from build123d import *

# Parameters (mm, degrees)
SKETCH_R        = 2.25
SKETCH_R_2      = 11.25
SKETCH_R_3      = 1.75
PAD_DEPTH       = 12
POCKET_DEPTH    = 9
SKETCH002_R     = 4
PAD001_DEPTH    = 9
SKETCH003_R     = 3
POCKET001_DEPTH = 8
SKETCH004_R     = 1.75
POCKET002_DEPTH = 10


with BuildPart() as pocket_belt_path:
    # Sketch → Pad (new body)
    with BuildSketch(Plane.XY):
        Polygon((0, 0), (105, 0), (105, 62), (20, 62), (20, 42), (0, 42), align=None)
        with Locations((35, 10)):
            Circle(SKETCH_R, mode=Mode.SUBTRACT)
        with Locations((30, 35)):
            Circle(SKETCH_R, mode=Mode.SUBTRACT)
        with Locations((84, 21)):
            Circle(SKETCH_R_2, mode=Mode.SUBTRACT)
        with Locations((68.5, 36.5)):
            Circle(SKETCH_R_3, mode=Mode.SUBTRACT)
        with Locations((99.5, 36.5)):
            Circle(SKETCH_R_3, mode=Mode.SUBTRACT)
        with Locations((68.5, 5.5)):
            Circle(SKETCH_R_3, mode=Mode.SUBTRACT)
        with Locations((99.5, 5.5)):
            Circle(SKETCH_R_3, mode=Mode.SUBTRACT)
        with Locations((10, 30)):
            Circle(SKETCH_R, mode=Mode.SUBTRACT)
        with Locations((10, 15)):
            Circle(SKETCH_R, mode=Mode.SUBTRACT)
        with Locations((39, 52)):
            Circle(SKETCH_R, mode=Mode.SUBTRACT)
        with Locations((94, 52)):
            Circle(SKETCH_R, mode=Mode.SUBTRACT)
        with Locations((55, 5)):
            Circle(SKETCH_R_3, mode=Mode.SUBTRACT)
    extrude(amount=PAD_DEPTH)

    # Sketch001 → Pocket (cut)
    with BuildSketch(Plane.XY.offset(12)):
        with BuildLine():
            ThreePointArc((38.485281, 42), (36.015595, 44.209377), (32.999996, 45.583006))
            Line((32.999996, 67), (32.999996, 45.583006))
            Line((20, 67), (32.999996, 67))
            Line((20, -1), (20, 67))
            Line((20, -1), (48.252269, -1))
            Line((48.252269, 11), (48.252269, -1))
            Line((48.252269, 11), (70.252269, 11))
            ThreePointArc((70.252269, 11), (71.759618, 9.202833), (73.499996, 7.630258))
            Line((73.499996, 7.630258), (73.499996, -1))
            Line((73.499996, -1), (93.499996, -1))
            Line((93.499996, -1), (93.499996, 6.902128))
            ThreePointArc((93.499996, 6.902128), (95.574295, 8.548671), (97.367695, 10.497399))
            Line((105.499996, 10.497399), (97.367695, 10.497399))
            Line((105.499996, 30.497399), (105.499996, 10.497399))
            Line((98.099621, 30.497399), (105.499996, 30.497399))
            ThreePointArc((98.099621, 30.497399), (91.98574, 36.007594), (83.999996, 38))
            Line((83.999996, 38), (83.999996, 67))
            Line((83.999996, 67), (43.999996, 67))
            Line((43.999996, 67), (43.999996, 42))
            Line((38.485281, 42), (43.999996, 42))
        make_face()
    extrude(amount=-POCKET_DEPTH, mode=Mode.SUBTRACT)


with BuildPart() as pocket002:
    # Part__Mirroring: instance of Pocket belt path
    add(pocket_belt_path.part.mirror(Plane(origin=(0, 0, 0), x_dir=(0, 1, 0), z_dir=(0, 0, 1))))

    # Sketch002 → Pad001 (new body)
    with BuildSketch(Plane(origin=(0, 0, -3), x_dir=(1, 0, 0), z_dir=(0, 0, -1))):
        with Locations((68.5, -36.5)):
            Circle(SKETCH002_R)
    extrude(amount=PAD001_DEPTH)

    # Sketch003 → Pocket001 (cut)
    with BuildSketch(Plane.XY):
        with Locations((55, 5)):
            Circle(SKETCH003_R)
        with Locations((68.5, 36.5)):
            Circle(SKETCH003_R)
        with Locations((68.5, 5.5)):
            Circle(SKETCH003_R)
        with Locations((99.5, 5.5)):
            Circle(SKETCH003_R)
        with Locations((99.5, 36.5)):
            Circle(SKETCH003_R)
    extrude(amount=-POCKET001_DEPTH, mode=Mode.SUBTRACT)

    # Sketch004 → Pocket002 (cut)
    with BuildSketch(Plane.XY.offset(-8)):
        with Locations((68.5, 36.5)):
            Circle(SKETCH004_R)
    extrude(amount=-POCKET002_DEPTH, mode=Mode.SUBTRACT)


with BuildPart() as part_mirroring001:
    # Part__Mirroring001: instance of Pocket002
    add(pocket002.part.mirror(Plane(origin=(0, 0, 0), x_dir=(0, -1, 0), z_dir=(1, 0, 0))))


solid = part_mirroring001.part
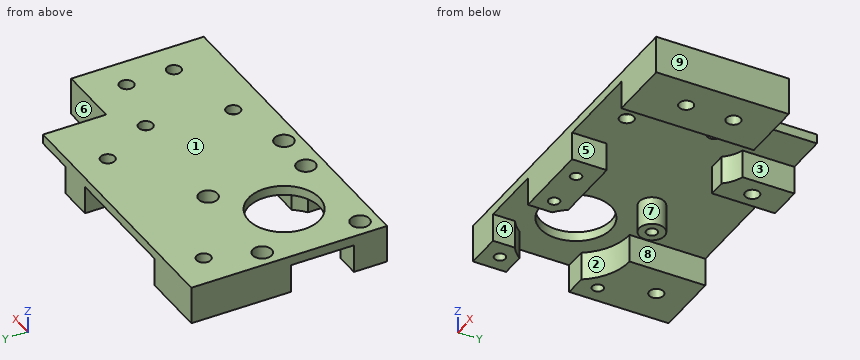
The listing builds one solid part. Answer for the finished solid, in the listing's coordinates (mm). Face numbers are marked on the shaded views. A direction names the side the tool comes from. Round coordinates to 2 decimals unless told otherwise and drop trailing zeros. Write each loop counter-clockwise with the first axis right and the second up, starting at its lowest first coordinate (ties: lowest second). Pieces come first, ordered by that corner, then holes. Notation, with made-up numbers: M 60.5,-24 L 86.5,-24 A29 ccw 86.5,13 Z; hole C 60.25,62.5 d3. An arc over 180 degrees is marked long. Write each question's results on one line, items separated by ' | '. Start each with the question number.
Item 1: For the marked faces 1, 2, 3, 4 and 5, determine the directions among +Z, -Z, +X, -X, +Y, -Y from which every point of the face is accessible in a straight line to the end or side of a thin tool.
Item 2: A cutting plane is placed at A-A on z = -4.25. State how many separate pieces and enclosed holes the cut face has, and give its area (3 significant figures).
Item 3: Flat-ended cylindrical pins translate along their axes: pin 1 Ø4.5 at (y, z) = (57, -6) entering from +X; pin 2 Ø4.5 at (x, z) = (-41.5, -8.5) entering from -Y; pin 3 Ø3 at (x, y) = (-99.5, 5.5) entering from +Z; pin 4 Ø3 at (x, y) = (-55.5, 5.5) entering from +Z. Find the tip coordinate at first contact, or state that the pin passes through.
Item 4: For a pull along X with two mould halves and no side action, classify the marked faces 6, 7, 8 and 9 as pulls with the +X half, pulls with the -X half, needs draft (parallel to the pull), parting line crosses it, or undercut.
Item 5: A cutting plane is placed at B-B on y = 52. Write down the section's boundary in (x, z), and give its area (3 significant figures).
Item 6: A cutting plane is placed at D-D on y = 21. Write down the section's boundary in (x, z).
Item 7: A cutting plane is placed at C-C on x = -99.5. Write down the section's boundary in (y, z), and give its area (3 significant figures).
Item 8: Straight lines are drawn through the part: L1, parallel to Y at x = -68.5, z = -9; L2, parallel to X at y = 46, z = -5.5; L3, parallel to Y at x = -9.5, z = -5.5. For each, find the intervals that lie inside material, in ascending order. Write a range as [from, to].
Check sheet entries:
1) face 1: +Z, +X, -X, +Y, -Y | face 2: -Z | face 3: -Z, +X, +Y, -Y | face 4: -Z, -Y | face 5: -Z, +Y, -Y
2) separate pieces: 6 | enclosed holes: 9 | area: 1,870 mm²
3) pin 1: x = -33 | pin 2: y = 42 | pin 3: through | pin 4: z = -8
4) face 6: needs draft | face 7: undercut | face 8: undercut | face 9: pulls with the +X half
5) outline: M -105,-12 L -96.25,-12 L -96.25,0 L -105,0 Z; M -91.75,-12 L -84,-12 L -84,-3 L -44,-3 L -44,-12 L -41.25,-12 L -41.25,0 L -91.75,0 Z; M -36.75,-12 L -33,-12 L -33,-3 L -20,-3 L -20,0 L -36.75,0 Z | area: 435 mm²
6) outline: M -105,-3 L -95.25,-3 L -95.25,0 L -105,0 Z; M -72.75,-3 L -20,-3 L -20,-12 L 0,-12 L 0,0 L -72.75,0 Z
7) outline: M 0,-12 L 3.75,-12 L 3.75,-8 L 2.5,-8 L 2.5,0 L 0,0 Z; M 7.25,-12 L 10.5,-12 L 10.5,-3 L 30.5,-3 L 30.5,-12 L 34.75,-12 L 34.75,-8 L 33.5,-8 L 33.5,0 L 8.5,0 L 8.5,-8 L 7.25,-8 Z; M 38.25,-12 L 62,-12 L 62,0 L 39.5,0 L 39.5,-8 L 38.25,-8 Z | area: 440 mm²
8) L1: [0, 3.75], [7.25, 11], [32.5, 34.75], [38.25, 40.5] | L2: [-105, -84], [-44, -33] | L3: [0, 12.81], [17.19, 27.81], [32.19, 42]
